Verification items for the finished model (mm, model axes). A direction names the side the tool comes from. Coordinates: 2 decimals unless noted, no trailing zeros. Loops run counter-clockwise (first coordinate to the right, second up) from the corner with the lowest first, then second, coordinate; pieces in that order, holes last. Notation, with made-up numbers: (-2, 30) -> (42, 30) arc R6 ccw to (42, 39) -> close; hole circle Ø3 at (80, -13). An arc over 180 degrees is marked (long way). Answer as a JSON object with one key per item and string values. Group by question number.
Q1. Release check for a two-part mould opening along Z. For faces 4 (the flat face through (-3.1, 9.1, 4.5)), 5 (the cylindrical face through (3.4, 11, -0.1)), 6 (the cylindrical face through (-1.31, 2.25, 0.02)) record: released by +Z, released by -Z, zero draft, split by the parting line, or undercut.
Q2. Set-up check for faces 1 (the cylindrical face through (0.59, 1.73, -4.46)), 2 (the flat face through (-2.85, 14, 0)), 3 (the flat face through (4.15, 12, 0)): record each of +Z, -Z, +X, -X, +Y, -Y from which the full face is reachable in a straight line by a thin tool's end or side.
Q3. Cross-section at C-C on y = 1.5. Record the boundary of the cut face in (x, z) (3 decimals), and give its area (3 significant figures).
Q4. Cross-section at A-A on y = 11. Record the boundary of the cut face in (x, z).
Q5. Gauge pin test, flat ends, axial feed: pin 1 Ø0.7 at (y, z) = (3, 1.5) entering from -X; pin 2 Ø0.8 at (y, z) = (14, 0.5) entering from +X; pin 3 Ø0.8 at (y, z) = (13.5, -2) entering from -X. Record the tip position at first contact, or that the pin passes through.
Q6. Scan lines: L1, parallel to X at y = 14, z = -0.25; L2, parallel to Y at x = 3, z = -3.25; L3, parallel to X at y = 9.75, z = 3.5. Record each from-to range of solid material in increasing order.
Q7. Cross-section at D-D on z = 0. Record the boundary of the cut face in (x, y), and give its area (3 significant figures).
Q8. Cross-section at B-B on x = 0. Record the boundary of the cut face in (y, z) (3 decimals).
Autodesk Inventor part; units mm, degrees
ref_plane "YZ Plane" through (0, 0, 0) normal (1, 0, 0) x (0, 1, 0)
ref_plane "XZ Plane" through (0, 0, 0) normal (0, 1, 0) x (-1, 0, 0)
ref_plane "XY Plane" through (0, 0, 0) normal (0, 0, 1) x (1, 0, 0)
sketch "Sketch1" plane through (0, 0, 0) normal (0, 1, 0) x (-1, 0, 0)
  circle A0 centre (0, 0) radius 1.05 construction
  arc A1 (-0.35, 1.2624) -> (-0.35, -1.2624) centre (0, 0) ccw
  circle A2 centre (0, 0) radius 4.5
  line L0 (0.35, 1.875) -> (-0.35, 1.875)
  line L1 (-0.35, 1.875) -> (-0.35, -1.875)
  line L2 (-0.35, -1.875) -> (0.35, -1.875)
  line L3 (0.35, -1.875) -> (0.35, 1.875)
  arc A3 (0.35, 1.2624) -> (-0.35, 1.2624) centre (0, 0) ccw
  arc A4 (0.35, -1.2624) -> (0.35, 1.2624) centre (0, 0) ccw
  arc A5 (-0.35, -1.2624) -> (0.35, -1.2624) centre (0, 0) ccw
  point P0 (0, 1.875)
  point P1 (0.35, 0)
  dimension "d1" = 2.1
  dimension "d3" = 9
  dimension "d18" = 0.26
  dimension "d19" = 0.7
  dimension "d20" = 3.75
extrude "Extrusion1" add sketch "Sketch1" along normal blind 3.5
sketch "Sketch4" plane through (0, 0, 0) normal (0, 0, 1) x (1, 0, 0)
  line L0 (-4.15, 15.5) -> (-4.15, 8.5)
  arc A0 (-4.15, 8.5) -> (4.15, 8.5) centre (0, 8.5) ccw
  line L1 (4.15, 8.5) -> (4.15, 15.5)
  line L2 (-2.85, 15.5) -> (-2.85, 12.854)
  arc A1 (-2.85, 8.5) -> (2.85, 8.5) centre (0, 8.5) ccw
  line L3 (2.85, 8.5) -> (2.85, 9.146)
  line L4 (-4.15, 15.5) -> (-2.85, 15.5)
  line L5 (2.85, 15.5) -> (4.15, 15.5)
  line L6 (-0.35, 0) -> (0.35, 0)
  line L7 (4.5, 3.5) -> (-4.5, 3.5)
  circle A2 centre (0, 11) radius 3.4
  line L8 (-2.85, 12.854) -> (-2.85, 9.146)
  line L9 (-2.85, 9.146) -> (-2.85, 8.5)
  line L10 (2.85, 9.146) -> (2.85, 12.854)
  line L11 (2.85, 12.854) -> (2.85, 15.5)
  point P0 (0, 0)
  point P1 (0, 0)
  dimension "d21" = 2.85
  dimension "d23" = 1.3
  dimension "d24" = 5
  dimension "d25" = 7
  dimension "d26" = 6.8
  dimension "d27" = 2.5
extrude "Extrusion5" add sketch "Sketch4" along normal mid plane 9 contours L4 L2 A2 L9 A1 L3 L11 L5 L1 A0 L0
sketch "Sketch8" plane through (0, 3.5, 0) normal (0, 1, 0) x (1, 0, 0)
  circle A0 centre (0, 0) radius 4
  arc A1 (0.35, -1.2624) -> (0.35, 1.2624) centre (0, 0) ccw
  line L0 (0.35, 1.875) -> (0.35, 1.2624)
  line L1 (-0.35, 1.875) -> (0.35, 1.875)
  line L2 (-0.35, 1.2624) -> (-0.35, 1.875)
  arc A2 (-0.35, 1.2624) -> (-0.35, -1.2624) centre (0, 0) ccw
  line L3 (-0.35, -1.875) -> (-0.35, -1.2624)
  line L4 (0.35, -1.875) -> (-0.35, -1.875)
  line L5 (0.35, -1.2624) -> (0.35, -1.875)
  dimension "d33" = 8
extrude "Extrusion6" add sketch "Sketch8" along normal up to next
sketch "Sketch2" plane through (0, 3.5, 0) normal (0, 1, 0) x (1, 0, 0)
  circle A0 centre (0, 0) radius 1.31
  circle A1 centre (0, 0) radius 3.31
  dimension "d6" = 2
  dimension "d9" = 7.3
  dimension "d10" = 2
properties part number "Laser Mount" material "ABS Plastic"
Computed values:
{
 "1": {"face 4": "released by +Z", "face 5": "zero draft", "face 6": "undercut"},
 "2": {"face 1": "-Y", "face 2": "+Z, -Z, +Y", "face 3": "+Z, -Z, +X, +Y"},
 "3": {"outline": "circle Ø9 at (0, 0); hole (-0.35, -1.875) -> (0.35, -1.875) -> (0.35, -1.262) arc R1.31 ccw to (0.35, 1.262) -> (0.35, 1.875) -> (-0.35, 1.875) -> (-0.35, 1.262) arc R1.31 ccw to (-0.35, -1.262) -> close", "area": "57.4 mm²"},
 "4": {"outline": "(-4.15, -4.5) -> (-3.4, -4.5) -> (-3.4, 4.5) -> (-4.15, 4.5) -> close; (3.4, -4.5) -> (4.15, -4.5) -> (4.15, 4.5) -> (3.4, 4.5) -> close"},
 "5": {"pin 1": "stops at x = -4.35", "pin 2": "stops at x = 4.15", "pin 3": "stops at x = -4.15"},
 "6": {"L1": "x = -4.15 to -2.85, 2.85 to 4.15", "L2": "y = 0 to 3.5, 5.63 to 9.4, 12.6 to 15.5", "L3": "x = -4.15 to -3.16, 3.16 to 4.15"},
 "7": {"outline": "(-4.5, 0) -> (-1.31, 0) -> (-1.31, 4.56) arc R4.15 ccw to (1.31, 4.56) -> (1.31, 0) -> (4.5, 0) -> (4.5, 3.5) -> (4, 3.5) -> (4, 7.39) arc R4.15 ccw to (4.15, 8.5) -> (4.15, 15.5) -> (2.85, 15.5) -> (2.85, 12.85) arc R3.4 cw to (2.85, 9.15) -> (2.85, 8.5) arc R2.85 cw to (-2.85, 8.5) -> (-2.85, 9.15) arc R3.4 cw to (-2.85, 12.85) -> (-2.85, 15.5) -> (-4.15, 15.5) -> (-4.15, 8.5) arc R4.15 ccw to (-4, 7.39) -> (-4, 3.5) -> (-4.5, 3.5) -> close", "area": "62.8 mm²"},
 "8": {"outline": "(0, -4.5) -> (3.5, -4.5) -> (3.5, -4) -> (4.35, -4) -> (4.35, -4.5) -> (5.65, -4.5) -> (5.65, 4.5) -> (4.35, 4.5) -> (4.35, 4) -> (3.5, 4) -> (3.5, 4.5) -> (0, 4.5) -> (0, 1.875) -> (4.35, 1.875) -> (4.35, -1.875) -> (0, -1.875) -> close"}
}
